from build123d import *

# Parameters (mm, degrees)
SKETCH_1_R          = 12
SKETCH_1_R_2        = 4.25
SKETCH_1_R_3        = 8
EXTRUDE_1_DEPTH     = 15
SKETCH_2_R          = 13.1
CUT_EXTRUDE_1_DEPTH = 10
CUT_EXTRUDE_2_REACH = 126
SKETCH_3_R          = 2.6
SKETCH_5_R          = 2.6
CUT_EXTRUDE_3_DEPTH = 10
SKETCH_6_W          = 50
SKETCH_6_H          = 50
CUT_EXTRUDE_4_DEPTH = 7
FILLET_1_R          = 2
FILLET_2_R          = 20


with BuildPart() as part:
    # Sketch 1 → Extrude 1 (new body)
    with BuildSketch(Plane.XY):
        Polygon((-33.800989673, 26.429197467), (-27.44059998, 26.429197467), (-18.800989673, 26.429197467), (-18.800989673, 10.718519348), (61.199010327, -69.281480652), (61.199010327, -82.570802533), (122.199010327, -82.570802533), (122.199010327, -18.570802533), (61.199010327, -18.570802533), (61.199010327, 26.429197467), (76.199010327, 26.429197467), (76.199010327, 41.429197467), (56.199010327, 41.429197467), (-33.800989673, 41.429197467), align=None)
        with Locations((41.199010327, 21.429197467)):
            Circle(SKETCH_1_R, mode=Mode.SUBTRACT)
        with Locations((46.199010327, -18.570802533)):
            Circle(SKETCH_1_R_2, mode=Mode.SUBTRACT)
        with Locations((91.699010327, -50.570802533)):
            Circle(SKETCH_1_R_3, mode=Mode.SUBTRACT)
        with BuildLine():
            Line((-11.034973369, 11.437784418), (2.9923212, 25.648765615))
            ThreePointArc((2.9923212, 25.648765615), (10.086164278, 25.671985824), (10.063536665, 18.57814083))
            Line((10.063536665, 18.57814083), (-4.055896558, 4.458707607))
            Line((-4.055896558, 4.458707607), (-11.034973369, 11.437784418))
        make_face(mode=Mode.SUBTRACT)
        with BuildLine():
            Line((106.999010327, -30.070802533), (106.999010327, -35.070802533))
            ThreePointArc((106.999010327, -35.070802533), (109.699010327, -37.770802533), (112.399010327, -35.070802533))
            Line((112.399010327, -35.070802533), (112.399010327, -30.070802533))
            ThreePointArc((112.399010327, -30.070802533), (109.699010327, -27.370802533), (106.999010327, -30.070802533))
        make_face(mode=Mode.SUBTRACT)
        with BuildLine():
            Line((70.999010327, -30.070802533), (70.999010327, -35.070802533))
            ThreePointArc((70.999010327, -35.070802533), (73.699010327, -37.770802533), (76.399010327, -35.070802533))
            Line((76.399010327, -35.070802533), (76.399010327, -30.070802533))
            ThreePointArc((76.399010327, -30.070802533), (73.699010327, -27.370802533), (70.999010327, -30.070802533))
        make_face(mode=Mode.SUBTRACT)
        with BuildLine():
            Line((76.399010327, -71.070802533), (76.399010327, -66.070802533))
            ThreePointArc((76.399010327, -66.070802533), (73.699010327, -63.370802533), (70.999010327, -66.070802533))
            Line((70.999010327, -66.070802533), (70.999010327, -71.070802533))
            ThreePointArc((70.999010327, -71.070802533), (73.699010327, -73.770802533), (76.399010327, -71.070802533))
        make_face(mode=Mode.SUBTRACT)
        with BuildLine():
            Line((112.399010327, -71.070802533), (112.399010327, -66.070802533))
            ThreePointArc((112.399010327, -66.070802533), (109.699010327, -63.370802533), (106.999010327, -66.070802533))
            Line((106.999010327, -66.070802533), (106.999010327, -71.070802533))
            ThreePointArc((106.999010327, -71.070802533), (109.699010327, -73.770802533), (112.399010327, -71.070802533))
        make_face(mode=Mode.SUBTRACT)
    extrude(amount=EXTRUDE_1_DEPTH)

    # Sketch 2 → Cut-Extrude 1 (cut)
    with BuildSketch(Plane(origin=(0, 0, 0), x_dir=(-1, 0, 0), z_dir=(0, 0, -1))):
        with Locations((-41.199010327, 21.429197467)):
            Circle(SKETCH_2_R)
    extrude(amount=-CUT_EXTRUDE_1_DEPTH, mode=Mode.SUBTRACT)

    # Sketch 3 → Cut-Extrude 2 (cut, up to next)
    with BuildSketch(Plane(origin=(0, 41.429197467, 0), x_dir=(1, 0, 0), z_dir=(0, 1, 0)), mode=Mode.PRIVATE) as cut_extrude_2_sk1:
        with Locations((-26.300989673, -7.5)):
            Circle(SKETCH_3_R)
    cut_extrude_2_tool1 = extrude(cut_extrude_2_sk1.sketch, amount=-CUT_EXTRUDE_2_REACH, mode=Mode.PRIVATE) & part.part
    add(cut_extrude_2_tool1.solids().sort_by_distance((-26.30099, 41.429197, 7.5))[0], mode=Mode.SUBTRACT)
    # Sketch 3 → Cut-Extrude 2 (cut, up to next)
    with BuildSketch(Plane(origin=(0, 41.429197467, 0), x_dir=(1, 0, 0), z_dir=(0, 1, 0)), mode=Mode.PRIVATE) as cut_extrude_2_sk2:
        with Locations((68.699010327, -7.5)):
            Circle(SKETCH_3_R)
    cut_extrude_2_tool2 = extrude(cut_extrude_2_sk2.sketch, amount=-CUT_EXTRUDE_2_REACH, mode=Mode.PRIVATE) & part.part
    add(cut_extrude_2_tool2.solids().sort_by_distance((68.69901, 41.429197, 7.5))[0], mode=Mode.SUBTRACT)

    # Sketch 5 → Cut-Extrude 3 (cut)
    with BuildSketch(Plane(origin=(-4.041235162, -4.041235162, 0), x_dir=(0, 0, 1), z_dir=(-0.707106781, -0.707106781, 0))):
        with Locations((7.5, 11.023445006)):
            Circle(SKETCH_5_R)
    extrude(amount=-CUT_EXTRUDE_3_DEPTH, mode=Mode.SUBTRACT)

    # Sketch 6 → Cut-Extrude 4 (cut)
    with BuildSketch(Plane(origin=(0, 0, 0), x_dir=(-1, 0, 0), z_dir=(0, 0, -1))):
        with Locations((-91.699010327, -50.570802533)):
            Rectangle(SKETCH_6_W, SKETCH_6_H)
    extrude(amount=-CUT_EXTRUDE_4_DEPTH, mode=Mode.SUBTRACT)

    # Fillet 1
    fillet_1_edges = [part.edges().sort_by_distance(p)[0] for p in [
        (116.699010327, -50.570802533, 7),
        (91.699010327, -25.570802533, 7),
        (66.699010327, -50.570802533, 7),
        (91.699010327, -75.570802533, 7),
    ]]
    fillet(fillet_1_edges, radius=FILLET_1_R)

    # Fillet 2
    fillet_2_edges = [part.edges().sort_by_distance(p)[0] for p in [
        (61.199010327, -18.570802533, 7.5),
    ]]
    fillet(fillet_2_edges, radius=FILLET_2_R)


solid = part.part
Source: CAD feature listing. Evaluate the final solid. Frame: model axes, mm. A direction names the side the tool comes from. Round coordinates to 2 decimals unless told otherwise and drop trailing zeros. Loops run counter-clockwise (first coordinate to the right, second up) from the corner with the lowest first, then second, coordinate; pieces in that order, holes last. Notation, with made-up numbers: (9.25, 13) - (45.25, 13) arc R22 cw to (45.25, 31) - close; hole circle Ø9 at (-18.5, 65.25). An arc over 180 degrees is marked (long way). Write item = value, one per line. Start each with the question number.
(1) Pull-direction query (Y, two-part tool) for faces 1 (the face through (20.64, -28.72, 7.4)), 2 (the face through (73.64, -73.77, 10.94)), 3 (the face through (-18.801, 19, 7)); classes: +Y half, -Y half, draft (parallel to the pull), parting line (faces both ways), or undercut.
(2) Ray query, line 1 along Y through (x, z) = (-9.5, 5.5); line 2 along X through (y, z) = (22.5, 4.5); line 3 along X through (y, z) = (30.5, 7.5). Return the intervals inside material, ascending. Write a range as from..to.
(3) Pin query (flat end, axial travel): pin 1 (4.5 mm diameter, centred on y = 17, z = 6.5, fed in from -X); pin 2 (23 mm diameter, centred on x = 81.5, y = -55.5, fed in from -Z); pin 3 (1.5 mm diameter, centred on x = 83.5, z = 3.5, fed in from +Y); pin 4 (7 mm diameter, centred on x = 46.2, y = -18.57, fed in from +Z). Return the tip coordinate at first contact, or that it passes through.
(4) Section query A-A, the plane y = -10.5. Output: boundary loops of the cut face in (x, z), plus the area to 3 significant figures.
(5) Set-up query: faces 4 (the face through (65, 26.429, 7)), 5 (the face through (29.6, 17.6, 10)), 6 (the face through (109.64, -73.77, 10.94)). Return all of +Z, -Z, +X, -X, +Y, -Y with unobstructed straight access to the full face (end or side cutting, diameter ignored); none if empty.
Conclusion:
q1.face_1 = -Y half
q1.face_2 = undercut
q1.face_3 = draft
q2.line_1 = 1.42..3.74, 8.44..9.9, 12.99..41.43
q2.line_2 = -18.8..-0.12, 11.54..28.14, 54.26..61.2
q2.line_3 = -33.8..-28.9, -23.7..31.75, 50.65..66.1, 71.3..76.2
q3.pin_1 = -18.8
q3.pin_2 = 7
q3.pin_3 = -18.57
q3.pin_4 = through
q4.outline = (2.42, 0) - (65.15, 0) - (65.15, 15) - (2.42, 15) - close
q4.area = 941 mm2
q5.face_4 = +Z, -Z, +X
q5.face_5 = -Z
q5.face_6 = +Z, -Z
